Can you work these out from the model? Positions are in its coordinate system, mm. Face numbers are marked on the shaded views. Round coordinates to 2 decimals unless told otherwise and drop trailing zeros. Write each loop counter-clockwise with the first axis right and the second up, starting at its lowest first coordinate (ties: lowest second). Pieces come first, ordered by that corner, then holes.
Q1. Please list where these lines run through material, in increasing order: line 1 along Z through (x, y) = (33.5, 11); line 2 along Z through (x, y) = (5, -1); line 3 along X through (y, z) = (-74, -4).
Q2. I'm going to push flat-ended pins straight in: pin 1 Ø9.5 at (x, z) = (-18.5, 19) entering from -Y; pin 2 Ø24 at (x, y) = (-13.5, -56.5) entering from +Z; pin 3 Ø5 at (x, z) = (2.5, -4.5) entering from -Y. Where does each tip first touch, or does it pass through?
Q3. We'd pull the mould along X, two halves only. Please class the marked faces 1, 2, 3 and 4: +X half, -X half, draft (parallel to the pull), parting line (faces both ways), or undercut.
Q4. If we section it at B-B (y = 31.5): Please give me the cut outline in (x, z), plus the area to 4 significant figures.
Q5. If we section it at C-C (z = 18.5): Please give me the cut outline in (x, y).
Q6. If we section it at A-A (x = 9.5): Please give me the cut outline in (y, z).
Q7. If we section it at D-D (y = -31): Please give me the cut outline in (x, z).
from build123d import *

# Parameters (mm, degrees)
F0_W     = 170
F0_H     = 3
F1_DEPTH = 52.5
F3_DEPTH = 40
F4_DEPTH = 40


with BuildPart() as f1:
    # F0 (on Right) → F1 (new body, symmetric)
    with BuildSketch(Plane.YZ):
        with BuildLine():
            ThreePointArc((-65, 21.5), (-79.142136, 15.642136), (-85, 1.5))
            Line((-85, 1.5), (85, 1.5))
            Line((85, 1.5), (85, 21.5))
            Line((85, 21.5), (-65, 21.5))
        make_face()
        with BuildLine():
            Line((85, -1.5), (-85, -1.5))
            ThreePointArc((-85, -1.5), (-79.142136, -15.642136), (-65, -21.5))
            Line((-65, -21.5), (85, -21.5))
            Line((85, -21.5), (85, -1.5))
        make_face()
        Rectangle(F0_W, F0_H)
    extrude(amount=F1_DEPTH, both=True)

    # F2 (on Right) → F3 (cut, symmetric)
    with BuildSketch(Plane.YZ):
        Polygon((0, 12.922657), (0, 22.922657), (-87.274782, 22.922657), (-84.384896, 12.922657), align=None)
    extrude(amount=F3_DEPTH, both=True, mode=Mode.SUBTRACT)

    # F2 (on Right) → F4 (cut, symmetric)
    with BuildSketch(Plane.YZ):
        Polygon((-75, -11.5), (75, -11.5), (75, 9.5), (-75, 9.5), (-75, 1.5), (-75, 0), (-75, -1.5), align=None)
        Polygon((0, 12.922657), (0, 22.922657), (-87.274782, 22.922657), (-84.384896, 12.922657), align=None)
    extrude(amount=F4_DEPTH, both=True, mode=Mode.SUBTRACT)


solid = f1.part
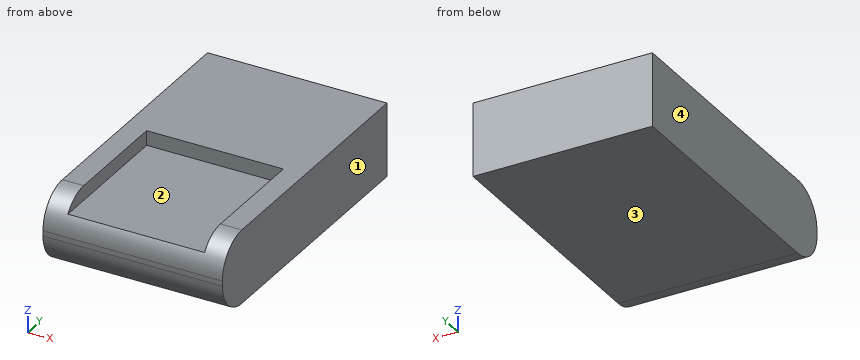
A:
1. line 1: z = -21.5 to -11.5, 9.5 to 21.5
1. line 2: z = -21.5 to -11.5, 9.5 to 12.92
1. line 3: x = -52.5 to -40, 40 to 52.5
2. pin 1: stops at y = 0
2. pin 2: stops at z = 12.92
2. pin 3: stops at y = -84.99
3. face 1: +X half
3. face 2: undercut
3. face 3: draft
3. face 4: -X half
4. outline: (-52.5, -21.5) - (52.5, -21.5) - (52.5, 21.5) - (-52.5, 21.5) - close; hole (-40, -11.5) - (40, -11.5) - (40, 9.5) - (-40, 9.5) - close
4. area: 2,835 mm2
5. outline: (-52.5, -75.54) - (-40, -75.54) - (-40, 0) - (40, 0) - (40, -75.54) - (52.5, -75.54) - (52.5, 85) - (-52.5, 85) - close
6. outline: (-85, -1.5) arc R20 ccw to (-65, -21.5) - (85, -21.5) - (85, 21.5) - (0, 21.5) - (0, 12.92) - (-81.42, 12.92) arc R20 ccw to (-85, 1.5) - close; hole (-75, -11.5) - (75, -11.5) - (75, 9.5) - (-75, 9.5) - close
7. outline: (-52.5, -21.5) - (52.5, -21.5) - (52.5, 21.5) - (40, 21.5) - (40, 12.92) - (-40, 12.92) - (-40, 21.5) - (-52.5, 21.5) - close; hole (-40, -11.5) - (40, -11.5) - (40, 9.5) - (-40, 9.5) - close
